```python
from build123d import *

# Parameters (mm, degrees)
SKETCH_1_W          = 80
SKETCH_1_H          = 60
SKETCH_1_W_2        = 47.3
SKETCH_1_H_2        = 47.3
EXTRUDE_1_DEPTH     = 8
SKETCH_2_R          = 5.5
SKETCH_2_R_2        = 1.55
SKETCH_2_W          = 12
SKETCH_2_H          = 20
CUT_EXTRUDE_1_DEPTH = 3.1
FILLET_1_R          = 1.5
SKETCH_3_R          = 1.55
CUT_EXTRUDE_2_DEPTH = 10
FILLET_2_R          = 8
SKETCH_4_R          = 3
CUT_EXTRUDE_3_DEPTH = 3.1
SKETCH_5_R          = 2.75
CUT_EXTRUDE_4_DEPTH = 10


with BuildPart() as part:
    # ｽｹｯﾁ1 → ﾎﾞｽ - 押し出し1 (new body)
    # profile 1 of 2: a face of its own
    with BuildSketch(Plane.XY):
        with Locations((23.65, 23.65)):
            Rectangle(SKETCH_1_W, SKETCH_1_H)
        with Locations((23.65, 23.65)):
            Rectangle(SKETCH_1_W_2, SKETCH_1_H_2, mode=Mode.SUBTRACT)
    # profile 2 of 2: a face of its own
    with BuildSketch(Plane.XY):
        with Locations((23.65, 23.65)):
            Rectangle(SKETCH_1_W_2, SKETCH_1_H_2)
    extrude(amount=EXTRUDE_1_DEPTH)

    # ｽｹｯﾁ2 → ｶｯﾄ - 押し出し1 (cut)
    with BuildSketch(Plane.XY.offset(8)):
        with Locations((23.65, 23.65)):
            Circle(SKETCH_2_R)
        with Locations((23.65, 35.15)):
            Circle(SKETCH_2_R_2)
        with Locations((5.65, 23.65)):
            Rectangle(SKETCH_2_W, SKETCH_2_H)
        with Locations((41.65, 23.65)):
            Rectangle(SKETCH_2_W, SKETCH_2_H)
    extrude(amount=-CUT_EXTRUDE_1_DEPTH, mode=Mode.SUBTRACT)

    # ﾌｨﾚｯﾄ1
    fillet_1_edges = [part.edges().sort_by_distance(p)[0] for p in [
        (11.65, 33.65, 6.45),
        (11.65, 13.65, 6.45),
        (-0.35, 13.65, 6.45),
        (-0.35, 33.65, 6.45),
        (47.65, 33.65, 6.45),
        (47.65, 13.65, 6.45),
        (35.65, 13.65, 6.45),
        (35.65, 33.65, 6.45),
    ]]
    fillet(fillet_1_edges, radius=FILLET_1_R)

    # ｽｹｯﾁ3 → ｶｯﾄ - 押し出し2 (cut)
    with BuildSketch(Plane.XY.offset(8)):
        with Locations((17.65, 40.65)):
            Circle(SKETCH_3_R)
        with Locations((29.65, 40.65)):
            Circle(SKETCH_3_R)
        with Locations((29.65, 6.65)):
            Circle(SKETCH_3_R)
        with Locations((17.65, 6.65)):
            Circle(SKETCH_3_R)
    extrude(amount=-CUT_EXTRUDE_2_DEPTH, mode=Mode.SUBTRACT)

    # ﾌｨﾚｯﾄ2
    fillet_2_edges = [part.edges().sort_by_distance(p)[0] for p in [
        (63.65, -6.35, 4),
        (-16.35, -6.35, 4),
        (-16.35, 53.65, 4),
        (63.65, 53.65, 4),
    ]]
    fillet(fillet_2_edges, radius=FILLET_2_R)

    # ｽｹｯﾁ4 → ｶｯﾄ - 押し出し3 (cut)
    with BuildSketch(Plane(origin=(0, 0, 0), x_dir=(-1, 0, 0), z_dir=(0, 0, -1))):
        with Locations((-29.65, 40.65)):
            Circle(SKETCH_4_R)
        with Locations((-17.65, 40.65)):
            Circle(SKETCH_4_R)
        with Locations((-17.65, 6.65)):
            Circle(SKETCH_4_R)
        with Locations((-29.65, 6.65)):
            Circle(SKETCH_4_R)
    extrude(amount=-CUT_EXTRUDE_3_DEPTH, mode=Mode.SUBTRACT)

    # ｽｹｯﾁ5 → ｶｯﾄ - 押し出し4 (cut)
    with BuildSketch(Plane.XY.offset(8)):
        with Locations((56.65, 0.65)):
            Circle(SKETCH_5_R)
        with Locations((56.65, 46.65)):
            Circle(SKETCH_5_R)
        with Locations((-9.35, 46.65)):
            Circle(SKETCH_5_R)
        with Locations((-9.35, 0.65)):
            Circle(SKETCH_5_R)
    extrude(amount=-CUT_EXTRUDE_4_DEPTH, mode=Mode.SUBTRACT)


solid = part.part
```
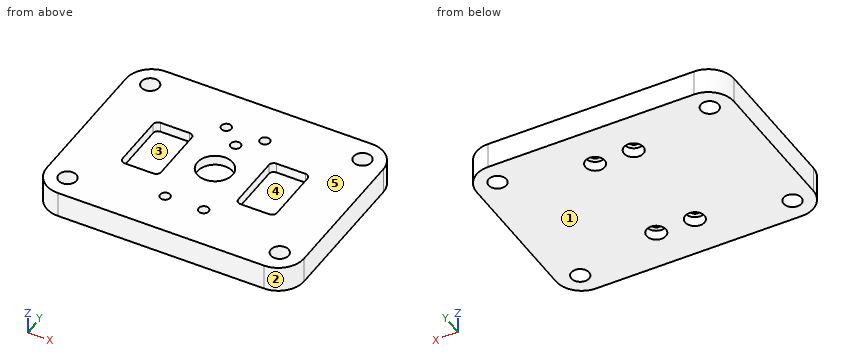
Source: CAD feature listing. Evaluate the final solid. Frame: model axes, mm. Face numbers are marked on the shaded views. A direction names the side the tool comes from. Round coordinates to 2 decimals unless told otherwise and drop trailing zeros. Loops run counter-clockwise (first coordinate to the right, second up) from the corner with the lowest first, then second, coordinate; pieces in that order, holes last. Notation, with made-up numbers: M 76,33 L 121,33 A19 ccw 121,70 Z; hole C -9,51.25 d2. An arc over 180 degrees is marked long. Put each result on its own line as item: value.
(1) Section D-D, the plane x = 58.5. Return loops of the section in (y, z), and give its area (3 significant figures).
Solutions:
outline: M -5.83,0 L -1.38,0 L -1.38,8 L -5.83,8 Z; M 2.68,0 L 44.62,0 L 44.62,8 L 2.68,8 Z; M 48.68,0 L 53.13,0 L 53.13,8 L 48.68,8 Z
area: 406 mm²
(2) Access query for the marked faces 4 and 5. Directions: +Z, -Z, +X, -X, +Y, -Y. A direction counts if a zero-diameter tool reaches every point of the face in a straight line with its end or side. Return the directions, or none.
Solutions:
face 4: +Z
face 5: +Z, +X, -X, +Y, -Y
(3) Ray query, line 1 (Y direction, x = 29.65, z = 1.45); line 2 (Y direction, x = 23.65, z = 5.65); line 3 (X direction, y = 46, z = 7.5). Return the intervals inside material, ascending. Write a range as [from, to].
Solutions:
line 1: [-6.35, 3.65], [9.65, 37.65], [43.65, 53.65]
line 2: [-6.35, 18.15], [29.15, 33.6], [36.7, 53.65]
line 3: [-16.34, -12.02], [-6.68, 53.98], [59.32, 63.64]
(4) Pull-direction query (X, two-part tool) for the marked faces 1, 2 and 3; classes: released by +X, released by -X, zero draft, split by the parting line, or undercut.
Solutions:
face 1: zero draft
face 2: released by +X
face 3: undercut
(5) Section A-A, the plane y = 6.65. Return loops of the section in (x, z), and give its area (3 significant figures).
Solutions:
outline: M -16.35,0 L 14.65,0 L 14.65,3.1 L 16.1,3.1 L 16.1,8 L -16.35,8 Z; M 19.2,3.1 L 20.65,3.1 L 20.65,0 L 26.65,0 L 26.65,3.1 L 28.1,3.1 L 28.1,8 L 19.2,8 Z; M 31.2,3.1 L 32.65,3.1 L 32.65,0 L 63.65,0 L 63.65,8 L 31.2,8 Z
area: 572 mm²
(6) First-contact query: pin 1 (1.9 mm diameter, centred on x = 17.65, y = 40.65, fed in from -Z); pin 2 (5 mm diameter, centred on x = 17.65, y = 6.65, fed in from -Z); pin 3 (5.5 mm diameter, centred on x = 22, y = 24.5, fed in from +Z). Flat tips, straight axial feed; report the tip coordinate or a pass-through.
Solutions:
pin 1: through
pin 2: z = 3.1
pin 3: z = 4.9
(7) Section C-C, the plane y = 23.65. Return loops of the section in (x, z).
Solutions:
outline: M -16.35,0 L 63.65,0 L 63.65,8 L 47.65,8 L 47.65,4.9 L 35.65,4.9 L 35.65,8 L 29.15,8 L 29.15,4.9 L 18.15,4.9 L 18.15,8 L 11.65,8 L 11.65,4.9 L -0.35,4.9 L -0.35,8 L -16.35,8 Z
(8) Section B-B, the plane x = 38. Return loops of the section in (y, z), and give its area (3 significant figures).
Solutions:
outline: M -6.35,0 L 53.65,0 L 53.65,8 L 33.65,8 L 33.65,4.9 L 13.65,4.9 L 13.65,8 L -6.35,8 Z
area: 418 mm²
